```python
from build123d import *

# Parameters (mm, degrees)
F0_W     = 114.3
F0_H     = 273.05
F1_DEPTH = 19.05
F2_W     = 3.175
F2_H     = 273.05
F3_DEPTH = 12.7
F5_DEPTH = 19.051


with BuildPart() as f1:
    # F0 (on Right) → F1 (new body)
    with BuildSketch(Plane.YZ):
        with Locations((-57.15, -136.525)):
            Rectangle(F0_W, F0_H)
    extrude(amount=F1_DEPTH)

    # F2 (on face) → F3 (cut)
    with BuildSketch(Plane.YZ.offset(19.05)):
        with Locations((-38.1, -136.525)):
            Rectangle(F2_W, F2_H)
        with Locations((-69.85, -136.525)):
            Rectangle(F2_W, F2_H)
        with Locations((-101.6, -136.525)):
            Rectangle(F2_W, F2_H)
    extrude(amount=-F3_DEPTH, mode=Mode.SUBTRACT)

    # F4 (on face) → F5 (cut, through all)
    with BuildSketch(Plane.YZ.offset(19.05)):
        Polygon((0, -193.016278), (-114.3, -273.05), (0, -273.05), align=None)
    extrude(amount=-F5_DEPTH, mode=Mode.SUBTRACT)


solid = f1.part
```
Can you work these out from the model? Positions are in its coordinate system, mm. A direction names the side the tool comes from. Coordinates: 2 decimals unless noted, no trailing zeros. Order: outer loops, then holes, each group sorted by start corner. A loop starts at its lowest first (then second) coordinate and runs counter-clockwise, first axis right, second up.
1. I'm going to push flat-ended pins straight in: pin 1 (1 mm diameter, centred on y = -38, z = -85, fed in from +X); pin 2 (2 mm diameter, centred on x = 9.5, y = -34.5, fed in from -Z); pin 3 (1 mm diameter, centred on x = 4, y = -100.5, fed in from -Z). Where does each tip first touch, or does it pass through?
2. If we section it at B-B (z = -150): Please give me the cut outline in (x, y), then the cut area to 3 significant figures.
3. Thinking about a two-plate mould opening in Y: for faces 3 (the face through (9, 0, -98)), 4 (the face through (19.05, -54, -119)), 5 (the face through (13, -39.688, -112)), 6 (the face through (9, -114.3, -138)), which applies, +Y half, -Y half, draft (parallel to the pull), parting line (faces both ways), or undercut?
4. For faces 1 (the face through (19.05, -109, -135)), 2 (the face through (13, -68.262, -122)), which set-ups out of +Z, -Z, +X, -X, +Y, -Y let a thin tool reach every point of the face, with its end or its side?
5. If we section it at C-C (y = -96.5): Please give me the cut outline in (x, z), then the cut area to 3 significant figures.
6. If we section it at A-A (x = 14): Please give me the cut outline in (y, z).
7. If we section it at D-D (z = -233.5): Please give me the cut outline in (x, y).
8. I need wall thicknesses on line 1 (Y direction, x = 10, z = -142.5); line 2 (Y direction, x = 9.75, z = -220); line 3 (Y direction, x = 17.5, z = -222.5). Which ranges of each line are inside material? Lowest first, please.
Entries:
1. pin 1: stops at x = 6.35
1. pin 2: stops at z = -217.87
1. pin 3: stops at z = -263.74
2. outline: (0, -114.3) - (19.05, -114.3) - (19.05, -103.19) - (6.35, -103.19) - (6.35, -100.01) - (19.05, -100.01) - (19.05, -71.44) - (6.35, -71.44) - (6.35, -68.26) - (19.05, -68.26) - (19.05, -39.69) - (6.35, -39.69) - (6.35, -36.51) - (19.05, -36.51) - (19.05, 0) - (0, 0) - close
2. area: 2,060 mm2
3. face 3: +Y half
3. face 4: draft
3. face 5: undercut
3. face 6: -Y half
4. face 1: +Z, -Z, +X, +Y, -Y
4. face 2: +Z, -Z, +X
5. outline: (0, -260.59) - (19.05, -260.59) - (19.05, 0) - (0, 0) - close
5. area: 4,960 mm2
6. outline: (-114.3, -273.05) - (-103.19, -265.27) - (-103.19, 0) - (-114.3, 0) - close; (-100.01, -263.05) - (-71.44, -243.04) - (-71.44, 0) - (-100.01, 0) - close; (-68.26, -240.81) - (-39.69, -220.81) - (-39.69, 0) - (-68.26, 0) - close; (-36.51, -218.58) - (0, -193.02) - (0, 0) - (-36.51, 0) - close
7. outline: (0, -114.3) - (19.05, -114.3) - (19.05, -103.19) - (6.35, -103.19) - (6.35, -100.01) - (19.05, -100.01) - (19.05, -71.44) - (6.35, -71.44) - (6.35, -68.26) - (19.05, -68.26) - (19.05, -57.82) - (0, -57.82) - close
8. line 1: y = -114.3 to -103.19, -100.01 to -71.44, -68.26 to -39.69, -36.51 to 0
8. line 2: y = -114.3 to -103.19, -100.01 to -71.44, -68.26 to -39.69
8. line 3: y = -114.3 to -103.19, -100.01 to -71.44, -68.26 to -42.11
